Read the model definition and answer for the solid it produces. Units are mm, in the model's axes. Face numbers are marked on the shaded views. A direction names the side the tool comes from. Coordinates: 2 decimals unless noted, no trailing zeros. Write each loop counter-clockwise with the first axis right and the second up, starting at its lowest first coordinate (ties: lowest second). Pieces come first, ordered by that corner, then holes. Notation, with made-up numbers: M 16.25,36 L 44.25,36 A10 cw 44.25,50 Z; hole C -24,27 d8. An arc over 180 degrees is marked long. Use a Markdown table: item, result. Add a question column.
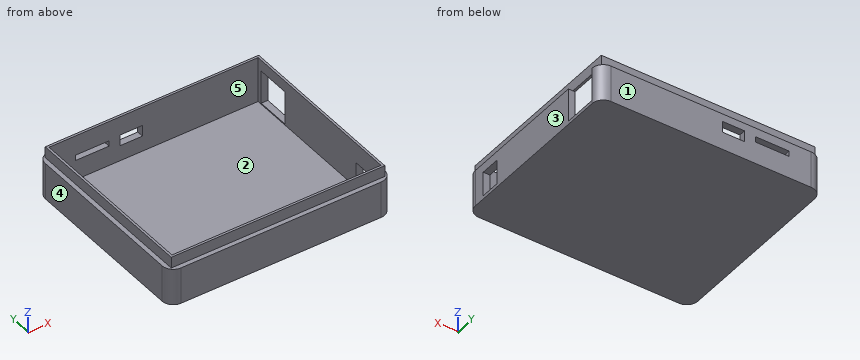
from build123d import *

# Parameters (mm, degrees)
SKETCH1_W           = 100
SKETCH1_H           = 85
BOSS_EXTRUDE2_DEPTH = 20
SKETCH3_W           = 100
SKETCH3_H           = 85
SKETCH3_W_2         = 96
SKETCH3_H_2         = 81
CUT_EXTRUDE1_DEPTH  = 5
SKETCH4_W           = 94
SKETCH4_H           = 79
CUT_EXTRUDE2_DEPTH  = 19
SKETCH9_W           = 100
SKETCH9_H           = 85
BOSS_EXTRUDE3_DEPTH = 1.5
SKETCH10_W          = 94
SKETCH10_H          = 79
CUT_EXTRUDE5_DEPTH  = 1.5
SKETCH11_W          = 11
SKETCH11_H          = 9
CUT_EXTRUDE7_DEPTH  = 50
SKETCH12_W          = 15
SKETCH12_H          = 15.24
CUT_EXTRUDE8_DEPTH  = 50
SKETCH13_W          = 15
SKETCH13_H          = 2.5
CUT_EXTRUDE9_DEPTH  = 50
SKETCH14_W          = 10
SKETCH14_H          = 5
CUT_EXTRUDE10_DEPTH = 50
FILLET1_R           = 5


with BuildPart() as part:
    # Sketch1 → Boss-Extrude2 (new body)
    with BuildSketch(Plane.XY):
        Rectangle(SKETCH1_W, SKETCH1_H)
    extrude(amount=BOSS_EXTRUDE2_DEPTH)

    # Sketch3 → Cut-Extrude1 (cut)
    with BuildSketch(Plane.XY.offset(20)):
        Rectangle(SKETCH3_W, SKETCH3_H)
        Rectangle(SKETCH3_W_2, SKETCH3_H_2, mode=Mode.SUBTRACT)
    extrude(amount=-CUT_EXTRUDE1_DEPTH, mode=Mode.SUBTRACT)

    # Sketch4 → Cut-Extrude2 (cut)
    with BuildSketch(Plane.XY.offset(20)):
        Rectangle(SKETCH4_W, SKETCH4_H)
    extrude(amount=-CUT_EXTRUDE2_DEPTH, mode=Mode.SUBTRACT)

    # Sketch9 → Boss-Extrude3 (add)
    with BuildSketch(Plane(origin=(0, 0, 0), x_dir=(-1, 0, 0), z_dir=(0, 0, -1))):
        Rectangle(SKETCH9_W, SKETCH9_H)
    extrude(amount=BOSS_EXTRUDE3_DEPTH)

    # Sketch10 → Cut-Extrude5 (cut)
    with BuildSketch(Plane.XY.offset(1)):
        Rectangle(SKETCH10_W, SKETCH10_H)
    extrude(amount=-CUT_EXTRUDE5_DEPTH, mode=Mode.SUBTRACT)

    # Sketch11 → Cut-Extrude7 (cut)
    with BuildSketch(Plane(origin=(50, 0, 0), x_dir=(0, 0, -1), z_dir=(1, 0, 0))):
        with Locations((-5.5, -28)):
            Rectangle(SKETCH11_W, SKETCH11_H)
    extrude(amount=-CUT_EXTRUDE7_DEPTH, mode=Mode.SUBTRACT)

    # Sketch12 → Cut-Extrude8 (cut)
    with BuildSketch(Plane(origin=(50, 0, 0), x_dir=(0, 0, -1), z_dir=(1, 0, 0))):
        with Locations((-7.5, 29.88)):
            Rectangle(SKETCH12_W, SKETCH12_H)
    extrude(amount=-CUT_EXTRUDE8_DEPTH, mode=Mode.SUBTRACT)

    # Sketch13 → Cut-Extrude9 (cut)
    with BuildSketch(Plane(origin=(0, 42.5, 0), x_dir=(1, 0, 0), z_dir=(0, 1, 0))):
        with Locations((-27.5, -9.75)):
            Rectangle(SKETCH13_W, SKETCH13_H)
    extrude(amount=-CUT_EXTRUDE9_DEPTH, mode=Mode.SUBTRACT)

    # Sketch14 → Cut-Extrude10 (cut)
    with BuildSketch(Plane(origin=(0, 42.5, 0), x_dir=(1, 0, 0), z_dir=(0, 1, 0))):
        with Locations((-10, -9)):
            Rectangle(SKETCH14_W, SKETCH14_H)
    extrude(amount=-CUT_EXTRUDE10_DEPTH, mode=Mode.SUBTRACT)

    # Fillet1
    fillet1_edges = [part.edges().sort_by_distance(p)[0] for p in [
        (50, -42.5, 6.75),
        (-50, -42.5, 6.75),
        (-50, 42.5, 6.75),
        (50, 42.5, 6.75),
    ]]
    fillet(fillet1_edges, radius=FILLET1_R)


solid = part.part
Item 1: For the marked faces 4 and 5, determine the directions among +Z, -Z, +X, -X, +Y, -Y from which every point of the face is accessible in a straight line to the end or side of a thin tool.
Item 2: Consider probe 1 along Y at (x, z) = (-19, 13.5); probe 2 along X at (y, z) = (-15.5, 1.25); probe 3 along X at (y, z) = (7, 15.75). Determine where each line is inside the solid, lowest interval first.
Item 3: Find section D-D on z = 18.5. Give the vertices of the cut face in (x, y), then the cut area to 3 significant figures.
Item 4: Find section C-C on x = -22.5. Give the vertices of the cut face in (y, z), then the cut area to 4 significant figures.
Item 5: Find section B-B on z = 2.5. Give the vertices of the cut face in (x, y), then the cut area to 3 significant figures.
Item 6: Find section A-A on y = 33. Give the vertices of the cut face in (x, z), then the cut area to 3 significant figures.
Item 7: Each of these flat-tipped pins is pushed along its axis until it touches: pin 1 (2.5 mm diameter, centred on y = 40.5, z = 8.5, fed in from +X); pin 2 (2.5 mm diameter, centred on x = 48, z = 3.5, fed in from +Y); pin 3 (12 mm diameter, centred on x = -34, y = 11.5, fed in from +Z); pin 4 (3.5 mm diameter, centred on x = -27.5, y = 41, fed in from +Z). Where does it stop, or does it pass through?
Item 8: Determine the mould class of the marked faces 1, 2 and 3 for opening direction Y: pulls with the +Y half, pulls with the -Y half, needs draft (parallel to the pull), parting line crosses it, or undercut.
Geometry says:
| question | item | result |
|---|---|---|
| 1 | face 4 | +Z, -Z, -X, +Y, -Y |
| 1 | face 5 | +Z |
| 2 | probe 1 | y = -42.5 to -39.5, 39.5 to 42.5 |
| 2 | probe 2 | x = -50 to -47, 47 to 50 |
| 2 | probe 3 | x = -48 to -47, 47 to 48 |
| 3 | outline | M -48,-40.5 L 48,-40.5 L 48,40.5 L -48,40.5 Z; hole M -47,-39.5 L 47,-39.5 L 47,39.5 L -47,39.5 Z |
| 3 | area | 350 mm2 |
| 4 | outline | M -42.5,-1.5 L 42.5,-1.5 L 42.5,8.5 L 39.5,8.5 L 39.5,-0.5 L -39.5,-0.5 L -39.5,20 L -40.5,20 L -40.5,15 L -42.5,15 Z; M 39.5,11 L 42.5,11 L 42.5,15 L 40.5,15 L 40.5,20 L 39.5,20 Z |
| 4 | area | 180.5 mm2 |
| 5 | outline | M -50,-37.5 A5 ccw -45,-42.5 L 45,-42.5 A5 ccw 50,-37.5 L 50,-32.5 L 47,-32.5 L 47,-39.5 L -47,-39.5 L -47,39.5 L 47,39.5 L 47,37.5 L 50,37.5 A5 ccw 45,42.5 L -45,42.5 A5 ccw -50,37.5 Z; M 47,-23.5 L 50,-23.5 L 50,22.26 L 47,22.26 Z |
| 5 | area | 980 mm2 |
| 6 | outline | M -50,-1.5 L 50,-1.5 L 50,0 L 47,0 L 47,-0.5 L -47,-0.5 L -47,20 L -48,20 L -48,15 L -50,15 Z; M 47,15 L 48,15 L 48,20 L 47,20 Z |
| 6 | area | 158 mm2 |
| 7 | pin 1 | stops at x = 49.68 |
| 7 | pin 2 | stops at y = 42.18 |
| 7 | pin 3 | stops at z = -0.5 |
| 7 | pin 4 | stops at z = 20 |
| 8 | face 1 | pulls with the +Y half |
| 8 | face 2 | undercut |
| 8 | face 3 | needs draft |
